Autodesk Inventor part; units mm, degrees
ref_plane "YZ Plane" through (0, 0, 0) normal (1, 0, 0) x (0, 1, 0)
ref_plane "XY Plane" through (0, 0, 0) normal (0, 0, 1) x (1, 0, 0)
sketch "Sketch1" plane through (0, 0, 0) normal (0, 0, 1) x (1, 0, 0)
  line L0 (-9.6047, -8) -> (9.6047, -8)
  line L1 (9.6047, 8) -> (-9.6047, 8)
  line L2 (0, 11.2) -> (0, -11.2)
  line L3 (-17.5, 0) -> (17.5, 0)
  arc A0 (-9.6047, 8) -> (-9.6047, -8) centre (0, 0) ccw
  arc A1 (9.6047, -8) -> (9.6047, 8) centre (0, 0) ccw
  point P0 (0, 0)
  point P1 (0, -8)
  point P2 (12.5, 0)
  point P3 (-12.5, 0)
  dimension "d0" = 16
  dimension "d15" = 12.5
  dimension "d16" = 12.5
  dimension "d17" = 25
  dimension "d19" = 8
extrude "Extrusion1" add sketch "Sketch1" along normal blind 3.2
sketch "Sketch2" plane through (0, 0, 3.2) normal (0, 0, 1) x (1, 0, 0)
  line L0 (0, 11.2) -> (0, -11.2)
  line L1 (-17.5, 0) -> (17.5, 0)
  circle A0 centre (0, 0) radius 4.575
  dimension "d4" = 9.15
extrude "Extrusion2" add sketch "Sketch2" along normal blind 2.6
sketch "Sketch3" plane through (0, 0, 5.8) normal (0, 0, 1) x (1, 0, 0)
  circle A0 centre (0, 0) radius 4.575
hole "Hole1" at (0, 0, 5.8) direction (0, 0, -1) diameter 6.647 end through all
fillet "Fillet1" radius 0.5 1 edges at (-4.575, 0, 3.2)
properties part number "20-081" material "Steel, Mild"
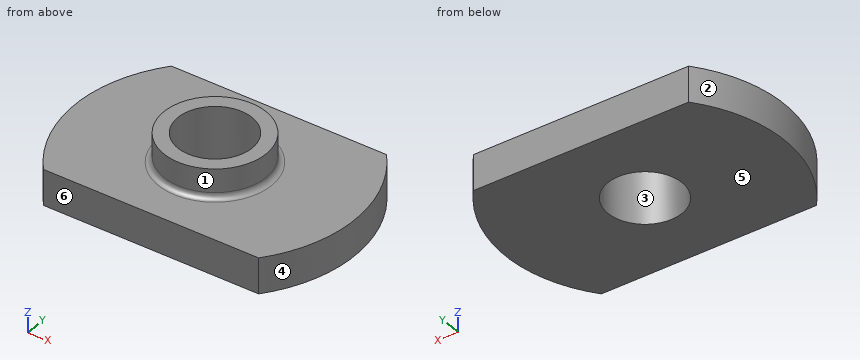
Input: part model. Units: mm. Frame: model coordinates. Face numbers are marked on the shaded views. A direction names the side the tool comes from. Coordinates: 2 decimals unless noted, no trailing zeros. Write each loop counter-clockwise with the first axis right and the second up, starting at its lowest first coordinate (ties: lowest second). Pieces come first, ordered by that corner, then holes. Notation, with made-up numbers: M 80,48.5 L 90,48.5 A30 ccw 90,84.5 Z; hole C 88,88.25 d9. An arc over 180 degrees is marked long. Use one line per item in the form item = value.
Q1. Section A-A (x = 0). Return loops of the section in (y, z) (1 decimal), plus the area to 3 significant figures.
Answer below:
outline = M -8,0 L -3.3,0 L -3.3,5.8 L -4.6,5.8 L -4.6,3.7 A0.5 cw -5.1,3.2 L -8,3.2 Z; M 3.3,0 L 8,0 L 8,3.2 L 5.1,3.2 A0.5 cw 4.6,3.7 L 4.6,5.8 L 3.3,5.8 Z
area = 36.5 mm²
Q2. Draft query along Y for the marked faces 3, 4, 5 and 6. Return one class per face: released by +Y, released by -Y, zero draft, split by the parting line, or undercut.
Answer below:
face_3 = undercut
face_4 = split by the parting line
face_5 = zero draft
face_6 = released by -Y
Q3. First-contact query: pin 1 (3 mm diameter, centred on x = -3.5, y = 5.5, fed in from +Z). Flat tip, straight axial feed; report the tip coordinate or a pass-through.
Answer below:
pin_1 = 3.2
Q4. Section B-B (y = 0). Return loops of the section in (x, z) (1 decimal), plus the area to 3 significant figures.
Answer below:
outline = M -12.5,0 L -3.3,0 L -3.3,5.8 L -4.6,5.8 L -4.6,3.7 A0.5 cw -5.1,3.2 L -12.5,3.2 Z; M 3.3,0 L 12.5,0 L 12.5,3.2 L 5.1,3.2 A0.5 cw 4.6,3.7 L 4.6,5.8 L 3.3,5.8 Z
area = 65.3 mm²
Q5. Material intervals for probe 1 along X at (y, z) = (0, 2.55); probe 2 along Y at (x, z) = (0, 2.8); probe 3 along Y at (x, z) = (0, 4.35) (1 decimal), sorted ascending. Write a range as from..to.
Answer below:
probe_1 = -12.5..-3.32, 3.32..12.5
probe_2 = -8..-3.32, 3.32..8
probe_3 = -4.6..-3.3, 3.3..4.6
Q6. Set-up query: the marked faces 1 and 2. Return all of +Z, -Z, +X, -X, +Y, -Y with unobstructed straight access to the full face (end or side cutting, diameter ignored); none if empty.
Answer below:
face_1 = +Z
face_2 = +Z, -Z, -X
Q7. Section C-C (z = 1.1). Return loops of the section in (x, y).
Answer below:
outline = M -9.6,-8 L 9.6,-8 A12.5 ccw 9.6,8 L -9.6,8 A12.5 ccw Z; hole C 0,0 d6.65
Q8. Section D-D (y = 6.25). Return loops of the section in (x, z).
Answer below:
outline = M -10.83,0 L 10.83,0 L 10.83,3.2 L -10.83,3.2 Z
